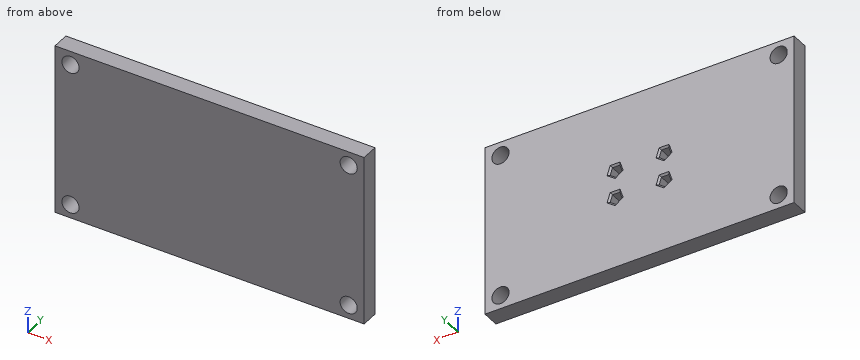
Autodesk Inventor part; units mm, degrees
ref_plane "YZ Plane" through (0, 0, 0) normal (1, 0, 0) x (0, 1, 0)
ref_plane "XZ Plane" through (0, 0, 0) normal (0, 1, 0) x (-1, 0, 0)
ref_plane "XY Plane" through (0, 0, 0) normal (0, 0, 1) x (1, 0, 0)
sketch "Sketch1" plane through (0, 0, 0) normal (0, 0, 1) x (1, 0, 0)
  line L0 (0, 0) -> (90, 0)
  line L1 (90, 0) -> (90, 5)
  line L2 (90, 5) -> (0, 5)
  line L3 (0, 5) -> (0, 0)
  dimension "d0" = 90
  dimension "d1" = 5
extrude "Extrusion1" add sketch "Sketch1" along normal blind 50
sketch "Sketch2" plane through (0, 5, 0) normal (0, 1, 0) x (1, 0, 0)
  line L0 (90, 0) -> (0, 0)
  line L1 (0, 0) -> (0, -50)
  line L2 (90, -50) -> (0, -50)
  line L3 (90, 0) -> (90, -50)
  line L4 (35, -18) -> (55, -18)
  line L5 (55, -18) -> (55, -32)
  line L6 (55, -32) -> (35, -32)
  line L7 (35, -32) -> (35, -18)
  line L8 (53.87, -28.5052) -> (53.2056, -30.55)
  line L9 (53.2056, -30.55) -> (51.0556, -30.55)
  line L10 (51.0556, -30.55) -> (50.3912, -28.5052)
  line L11 (50.3912, -28.5052) -> (52.1306, -27.2415)
  line L12 (52.1306, -27.2415) -> (53.87, -28.5052)
  line L13 (37.8694, -27.2415) -> (39.6088, -28.5052)
  line L14 (39.6088, -28.5052) -> (38.9444, -30.55)
  line L15 (38.9444, -30.55) -> (36.7944, -30.55)
  line L16 (36.7944, -30.55) -> (36.13, -28.5052)
  line L17 (36.13, -28.5052) -> (37.8694, -27.2415)
  line L18 (37.8694, -19.1) -> (39.6088, -20.3637)
  line L19 (39.6088, -20.3637) -> (38.9444, -22.4085)
  line L20 (38.9444, -22.4085) -> (36.7944, -22.4085)
  line L21 (36.7944, -22.4085) -> (36.13, -20.3637)
  line L22 (36.13, -20.3637) -> (37.8694, -19.1)
  line L23 (52.1306, -19.1) -> (53.87, -20.3637)
  line L24 (53.87, -20.3637) -> (53.2056, -22.4085)
  line L25 (53.2056, -22.4085) -> (51.0556, -22.4085)
  line L26 (51.0556, -22.4085) -> (50.3912, -20.3637)
  line L27 (50.3912, -20.3637) -> (52.1306, -19.1)
  point P0 (52.1306, -29.0704)
  point P1 (37.8694, -29.0704)
  point P2 (37.8694, -20.9289)
  point P3 (52.1306, -20.9289)
  point P4 (52.1306, -22.4085)
  dimension "d4" = 20
  dimension "d5" = 14
  dimension "d6" = 18
  dimension "d7" = 18
  dimension "d8" = 35
  dimension "d9" = 35
  dimension "d11" = 1.13
  dimension "d12" = 1.45
  dimension "d13" = 1.45
  dimension "d15" = 1.13
  dimension "d16" = 1.13
  dimension "d17" = 1.1
  dimension "d18" = 1.1
  dimension "d19" = 1.13
  dimension "d28" = 2.15
  dimension "d29" = 2.15
  dimension "d30" = 4.833
  dimension "d31" = 2.15
  dimension "d32" = 2.15
  dimension "d33" = 4.833
extrude "Extrusion2" cut sketch "Sketch2" against normal blind 4.5 contours L8 L9 L10 L11 L12 | L13 L14 L15 L16 L17 | L18 L19 L20 L21 L22 | L23 L24 L25 L26 L27
chamfer "Chamfer1" distance 0.5 angle 45 20 edges at (36.9997, 5, 27.8734) (36.4622, 5, 29.5276) (37.8694, 5, 30.55) (39.2766, 5, 29.5276) (38.7391, 5, 27.8734) (36.9997, 5, 19.7319) (36.4622, 5, 21.3861) (37.8694, 5, 22.4085) (39.2766, 5, 21.3861) (38.7391, 5, 19.7319) (50.7234, 5, 29.5276) (51.2609, 5, 27.8734) (53.0003, 5, 27.8734) (53.5378, 5, 29.5276) (52.1306, 5, 30.55) (52.1306, 5, 22.4085) (50.7234, 5, 21.3861) (51.2609, 5, 19.7319) (53.5378, 5, 21.3861) (53.0003, 5, 19.7319)
sketch "Sketch3" plane through (0, 5, 0) normal (0, 1, 0) x (1, 0, 0)
  line L0 (90, 0) -> (0, 0)
  line L1 (90, -50) -> (0, -50)
  line L2 (90, 0) -> (90, -50)
  line L3 (0, 0) -> (0, -50)
  point P0 (4.5, -46)
  point P1 (4.5, -4)
  point P2 (85.5, -46)
  point P3 (85.5, -4)
  dimension "d46" = 4.5
  dimension "d47" = 4.5
  dimension "d48" = 4
  dimension "d49" = 4
  dimension "d57" = 4.5
  dimension "d58" = 4.5
  dimension "d59" = 4
  dimension "d60" = 4
hole "Hole2" at (4.5, 5, 46) at (4.5, 5, 4) at (85.5, 5, 4) at (85.5, 5, 46) direction (0, -1, 0) diameter 5 end through all
properties part number "Hoofdplaat onderkant"
Build history of the part. All positions in model axes, mm. Give positions to 0.01 mm unless a question says otherwise; leave off trailing zeros. Loops run counter-clockwise (first coordinate to the right, second up) from the corner with the lowest first, then second, coordinate; pieces in that order, holes last.
Item 1: Slice it at B-B, the plane z = 4. List the corners of the cut face in (x, y), and give its area (3 significant figures).
Answers follow:
outline: (0, 0) - (2, 0) - (2, 5) - (0, 5) - close; (7, 0) - (83, 0) - (83, 5) - (7, 5) - close; (88, 0) - (90, 0) - (90, 5) - (88, 5) - close
area: 400 mm2
Item 2: Flat gauge pin, fed straight in: pin 1 (2.5 mm diameter, centred on x = 38, z = 29.5, fed in from +Y). Where does the tip first touch, or does it go through?
Answers follow:
pin 1: stops at y = 4.7
Item 3: Drill centre lines: line 1 (X direction, y = 1.75, z = 4); line 2 (Z direction, x = 85.5, y = 3); line 3 (X direction, y = 1.7, z = 3.5). Where is each one in solid material? Low to high.
Answers follow:
line 1: x = 0 to 2, 7 to 83, 88 to 90
line 2: z = 0 to 1.5, 6.5 to 43.5, 48.5 to 50
line 3: x = 0 to 2.05, 6.95 to 83.05, 87.95 to 90
Item 4: Slice it at A-A, the plane x = 84. List the corners of the cut face in (y, z), and give its area (3 significant figures).
Answers follow:
outline: (0, 0) - (5, 0) - (5, 2) - (0, 2) - close; (0, 6) - (5, 6) - (5, 44) - (0, 44) - close; (0, 48) - (5, 48) - (5, 50) - (0, 50) - close
area: 210 mm2
Item 5: Slice it at C-C, the plane y = 2.6. Give the number of separate pieces and of enclosed holes in the cut face, and give its area (3 significant figures).
Answers follow:
separate pieces: 1
enclosed holes: 8
area: 4,390 mm2
